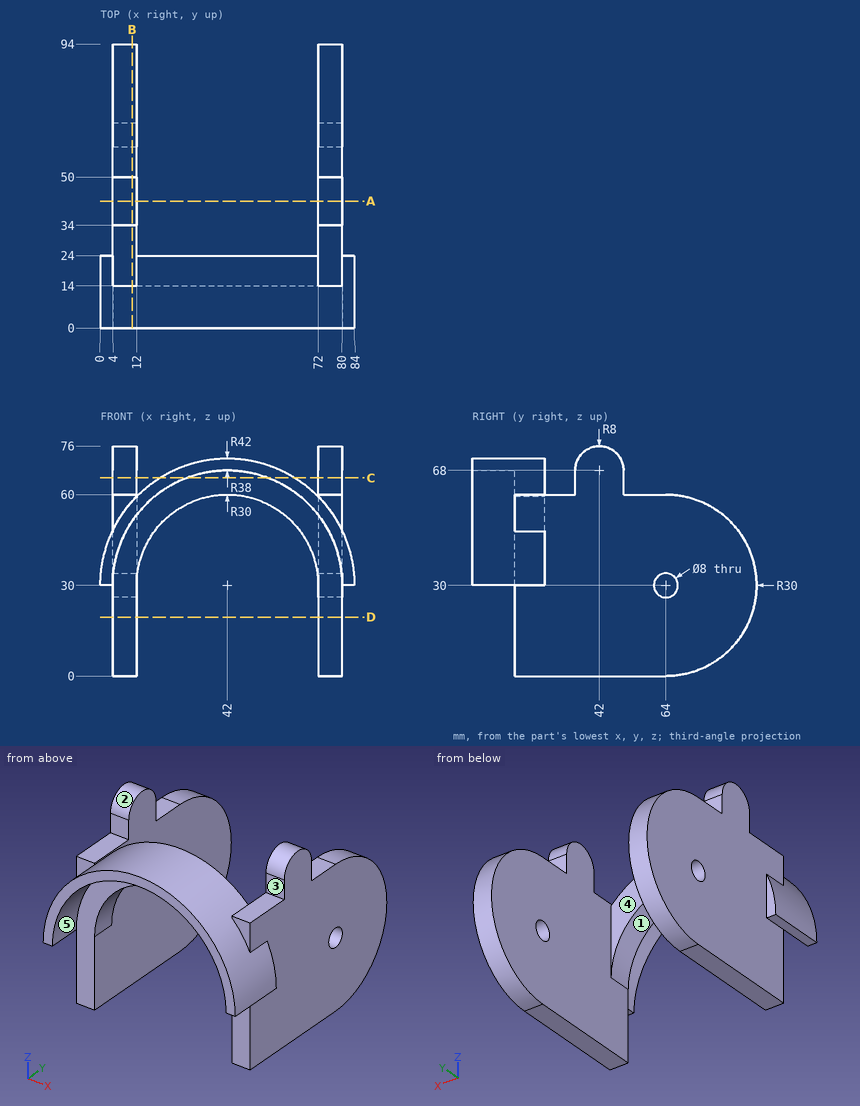
Design review of the part shown in the three views and the two pictorial views. Dimensions are in mm from the part's minimum x, y and z. A direction names the side the tool comes from. Round coordinates to 2 decimals unless told otherwise and drop trailing zeros. Loops run counter-clockwise (first coordinate to the right, second up) from the corner with the lowest first, then second, coordinate; pieces in that order, holes last. Notation, with made-up numbers: (-16, 17) -> (12, 17) arc R25 cw to (12, 31) -> close; hole circle Ø4 at (27.5, 76). An arc over 180 degrees is marked (long way). Use one line per item in the form item = value. Start each with the question number.
Q1. We need section D-D on z = 19.5. Give the boundary of the cut face in (x, y), then the cut area to 3 significant figures.
Q2. Wall thickness on line 1 along X through (y, z) = (16.5, 10.5); line 2 along Y through (x, z) = (76, 30); line 3 along Y through (x, z) = (51.5, 69): over which ranges is each line inside the solid? List them lowest first. Write a range as [from, to].
Q3. We need section C-C on z = 65.5. Give the boundary of the cut face in (x, y).
Q4. We need section A-A on y = 42. Give the boundary of the cut face in (x, z), then the cut area to 3 significant figures.
Q5. For pin 1 Ø8 at (y, z) = (38, 51.5) entering from +X; pin 2 Ø8 at (x, z) = (8.5, 30.5) entering from -Y; pin 3 Ø2.5 at (x, y) = (9.5, 55.5) entering from +Z, all flat-tipped, find the tip position at first contact; note any pin that passes through.
Q6. Machinability: for the marked faces 1, 2, 3, 4 and 5, which of the approach directions +Z, -Z, +X, -X, +Y, -Y give a long, thin tool a straight path to every point of the face, cutting with its end or side? Answer none if there is none.
Q7. We need section B-B on x = 10.5. Give the boundary of the cut face in (y, z), then the cut area to 3 significant figures.
Calculated:
q1.outline = (4, 14) -> (12, 14) -> (12, 92.1) -> (4, 92.1) -> close; (72, 14) -> (80, 14) -> (80, 92.1) -> (72, 92.1) -> close
q1.area = 1,250 mm²
q2.line_1 = [4, 12], [72, 80]
q2.line_2 = [14, 60], [68, 94]
q2.line_3 = [0, 24]
q3.outline = (4, 34) -> (12, 34) -> (12, 50) -> (4, 50) -> close; (19.56, 0) -> (28.44, 0) -> (28.44, 14) -> (55.56, 14) -> (55.56, 0) -> (64.44, 0) -> (64.44, 24) -> (19.56, 24) -> close; (72, 34) -> (80, 34) -> (80, 50) -> (72, 50) -> close
q4.outline = (4, 0) -> (12, 0) -> (12, 76) -> (4, 76) -> close; (72, 0) -> (80, 0) -> (80, 76) -> (72, 76) -> close
q4.area = 1,220 mm²
q5.pin_1 = 80
q5.pin_2 = 14
q5.pin_3 = 60
q6.face_1 = -Z, +Y, -Y
q6.face_2 = +Z, +X, -X
q6.face_3 = +Z, +X, -X, -Y
q6.face_4 = +Z, -Z, +Y
q6.face_5 = -Z, -Y
q7.outline = (0, 51.25) -> (14, 51.25) -> (14, 0) -> (64, 0) arc R30 ccw to (64, 60) -> (50, 60) -> (50, 68) arc R8 ccw to (34, 68) -> (34, 60) -> (14, 60) -> (14, 57.78) -> (0, 57.78) -> close; hole circle Ø8 at (64, 30)
q7.area = 4,680 mm²
